Input: dimensioned drawing with shaded views. Units: mm. Origin: part minimum x, y, z. A direction names the side the tool comes from. Round coordinates to 2 decimals unless told otherwise and drop trailing zeros. Loops run counter-clockwise (first coordinate to the right, second up) from the corner with the lowest first, then second, coordinate; pieces in that order, holes last. Notation, with made-up numbers: M -7.75,-25 L -1.75,-25 A26 ccw -1.75,4 Z; hole C -11,22.25 d2. An arc over 180 degrees is marked long. Return JSON: item names as keys, results as strings.
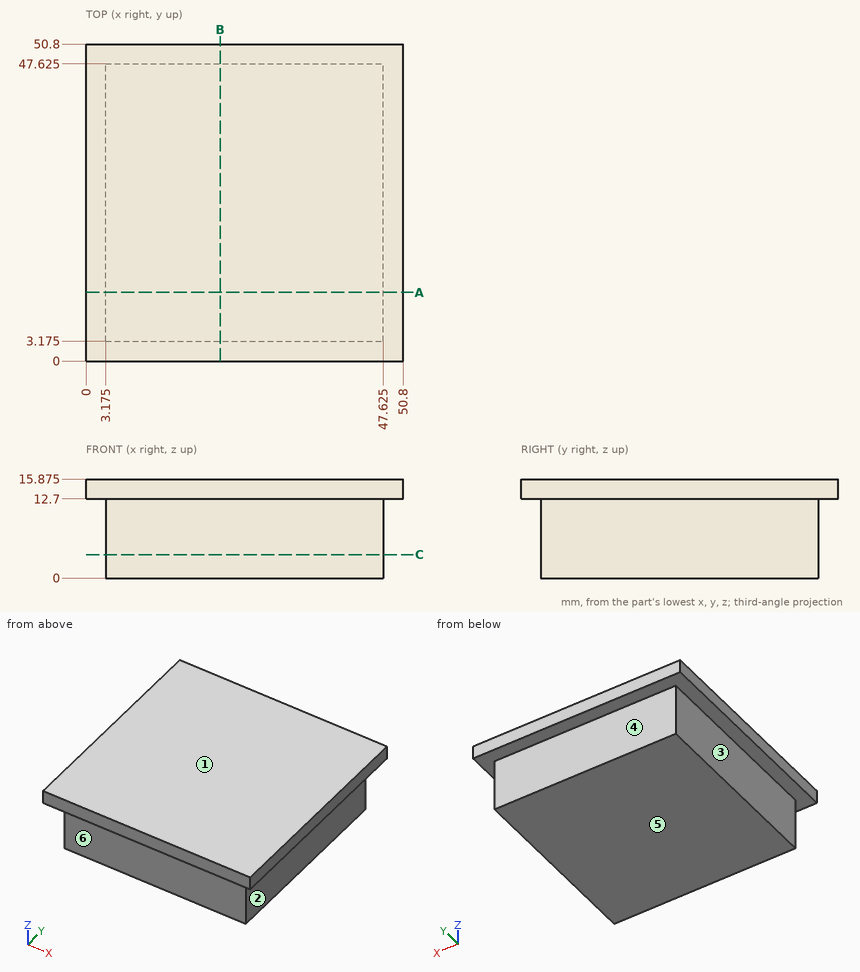
Q1. Section query A-A (y = 11). Output: boundary loops of the cut face in (x, z) (3 decimals), plus the area to 3 significant figures.
Determined:
{"outline": "M 0,12.7 L 3.175,12.7 L 3.175,0 L 47.625,0 L 47.625,12.7 L 50.8,12.7 L 50.8,15.875 L 0,15.875 Z", "area": "726 mm^2"}
Q2. Pin query (flat end, axial travel): pin 1 (4 mm diameter, centred on x = 25.5, z = 8.5, fed in from +Y) (3 decimals); pin 2 (6.5 mm diameter, centred on y = 24.5, z = 8.5, fed in from -X) (3 decimals); pin 3 (6.5 mm diameter, centred on x = 35.5, z = 8.5, fed in from -Y) (3 decimals). Return the tip coordinate at first contact, or that it passes through.
Determined:
{"pin 1": "stops at y = 47.625", "pin 2": "stops at x = 3.175", "pin 3": "stops at y = 3.175"}
Q3. Material intervals for L1, parallel to Y at x = 24.5, z = 3.75 (3 decimals); L2, parallel to Z at x = 37, y = 48 (3 decimals), sorted ascending.
Determined:
{"L1": "y = 3.175 to 47.625", "L2": "z = 12.7 to 15.875"}
Q4. Pull-direction query (X, two-part tool) for the marked faces 1, 2 and 3; classes: pulls with the +X half, pulls with the -X half, needs draft (parallel to the pull), parting line crosses it, or undercut.
Determined:
{"face 1": "needs draft", "face 2": "pulls with the +X half", "face 3": "pulls with the -X half"}
Q5. Reachability of the marked faces 4, 5 and 6 from +Z, -Z, +X, -X, +Y, -Y: full face, straight path, thin tool, end or side. Return the list, or none.
Determined:
{"face 4": "-Z, +X, -X, +Y", "face 5": "-Z, +X, -X, +Y, -Y", "face 6": "-Z, +X, -X, -Y"}
Q6. Section query C-C (z = 3.75). Output: boundary loops of the cut face in (x, y) (3 decimals), plus the area to 3 significant figures.
Determined:
{"outline": "M 3.175,3.175 L 47.625,3.175 L 47.625,47.625 L 3.175,47.625 Z", "area": "1,980 mm^2"}
